from build123d import *

# Parameters (mm, degrees)
SALIENTE_EXTRUIR1_DEPTH = 11
REDONDEO1_R             = 5
REDONDEO2_R             = 3
CROQUIS2_R              = 2.5
SALIENTE_EXTRUIR2_DEPTH = 11
CROQUIS3_W              = 8
CROQUIS3_H              = 15
CORTAR_EXTRUIR1_DEPTH   = 15
CROQUIS4_W              = 1.857543752
CROQUIS4_H              = 12.596468565
SALIENTE_EXTRUIR3_DEPTH = 13


with BuildPart() as part:
    # Croquis1 → Saliente-Extruir1 (new body)
    with BuildSketch(Plane.XY):
        Polygon((0, 9.6), (0, -9.6), (-32, -9), (-32, 9), align=None)
    extrude(amount=SALIENTE_EXTRUIR1_DEPTH)

    # Redondeo1
    redondeo1_edges = [part.edges().sort_by_distance(p)[0] for p in [
        (-32, -9, 5.5),
        (-32, 9, 5.5),
    ]]
    fillet(redondeo1_edges, radius=REDONDEO1_R)

    # Redondeo2
    redondeo2_edges = [part.edges().sort_by_distance(p)[0] for p in [
        (-13.546866762, 9.345996248, 11),
        (-13.546866762, -9.345996248, 0),
        (-13.546866762, -9.345996248, 11),
        (-32, 0, 0),
        (-30.568519835, 7.595108483, 0),
        (-30.568519835, -7.595108483, 0),
        (-32, 0, 11),
        (-30.568519835, 7.595108483, 11),
        (-30.568519835, -7.595108483, 11),
        (-13.546866762, 9.345996248, 0),
    ]]
    fillet(redondeo2_edges, radius=REDONDEO2_R)

    # Croquis2 → Saliente-Extruir2 (add)
    with BuildSketch(Plane.ZY.offset(32)):
        with Locations((5.5, 0)):
            Circle(CROQUIS2_R)
    extrude(amount=SALIENTE_EXTRUIR2_DEPTH)

    # Croquis3 → Cortar-Extruir1 (cut)
    with BuildSketch(Plane(origin=(0, 0, 0), x_dir=(0, 0, -1), z_dir=(1, 0, 0))):
        with Locations((-5.5, 0)):
            Rectangle(CROQUIS3_W, CROQUIS3_H)
    extrude(amount=-CORTAR_EXTRUIR1_DEPTH, mode=Mode.SUBTRACT)

    # Croquis4 → Saliente-Extruir3 (add)
    with BuildSketch(Plane(origin=(-15, 0, 0), x_dir=(0, 0, -1), z_dir=(1, 0, 0))):
        with Locations((-6.633221346, -0.002349923)):
            Rectangle(CROQUIS4_W, CROQUIS4_H)
    extrude(amount=SALIENTE_EXTRUIR3_DEPTH)


solid = part.part
Can you work these out from the model? Positions are in its coordinate system, mm. A direction names the side the tool comes from. Coordinates: 2 decimals unless noted, no trailing zeros. Loops run counter-clockwise (first coordinate to the right, second up) from the corner with the lowest first, then second, coordinate; pieces in that order, holes last. Notation, with made-up numbers: (41.25, 54.25) - (78.25, 54.25) arc R13 ccw to (78.25, 62.25) - close; hole circle Ø3 at (-23.5, 29.25). An arc over 180 degrees is marked (long way). Answer as a JSON object with one key per item and string values. Group by question number.
Item 1: If I drill on L1, parallel to Z at x = -6, y = -5; L2, parallel to Y at x = -7, z = 6; L3, parallel to Y at x = -7, z = 3.5, over which ranges is the centre line in solid material (lowest first)? Write a range as from..to.
Item 2: If we mould it in two halves opening along Z, with no side actions, what happens to faces 4 (the face through (-14, 0, 0)), 5 (the face through (-2, 0, 7)), 6 (the face through (-43, 0, 5))? For each: released by +Z, released by -Z, zero draft, split by the parting line, or undercut.
Item 3: For pin 1 (2.5 mm diameter, centred on x = -9, z = 4.5, fed in from +Y); pin 2 (5 mm diameter, centred on y = 7.5, z = 2.5, fed in from -X); pin 3 (2 mm diameter, centred on x = -11, z = 6.5, fed in from -Y); pin 4 (5 mm diameter, centred on x = -37, y = 6, fed in from -Z), each with a flat end and sliding along its axis, tell me the tip position at first contact or that it passes through.
Item 4: On a 3-axis mill with a long thin cutter (end or side, diameter ignored), from which of +Z, -Z, +X, -X, +Y, -Y can I reach the whole of each face in a straight line? I mean faces 1 (the face through (-13.34, 8.49, 0.9)), 2 (the face through (-9, 0, 7.562)), 3 (the face through (-13.72, -8.44, 10.145)). Say none if no direction works.
Item 5: If we section it at B-B (x = -9): State how many separate pieces and enclosed holes the cut face has, plus the area to 3 significant figures.
Item 6: If we section it at A-A (y = 1.5): List the corners of the cut face in (x, z) for me, plus the area to 3 significant figures.
Item 7: If we section it at D-D (x = -38.5): List the corners of the cut face in (y, z) for me.
Item 8: If we section it at C-C (z = 6.5): List the corners of the cut face in (x, y) for me, plus the area to 3 significant figures.
Returned:
{
 "1": {"L1": "z = 0..1.5, 5.7..7.56, 9.5..11", "L2": "y = -9.47..-7.5, -6.3..6.3, 7.5..9.47", "L3": "y = -9.47..-7.5, 7.5..9.47"},
 "2": {"face 4": "released by -Z", "face 5": "undercut", "face 6": "zero draft"},
 "3": {"pin 1": "stops at y = 9.45", "pin 2": "stops at x = -31.91", "pin 3": "stops at y = -9.41", "pin 4": "passes through"},
 "4": {"face 1": "-Z, -X, +Y", "face 2": "+X", "face 3": "+Z, -X, -Y"},
 "5": {"separate pieces": "2", "enclosed holes": "1", "area": "103 mm²"},
 "6": {"outline": "(-43, 3.5) - (-32, 3.5) - (-32, 3) arc R3 ccw to (-29, 0) - (0, 0) - (0, 1.5) - (-15, 1.5) - (-15, 5.7) - (-2, 5.7) - (-2, 7.56) - (-15, 7.56) - (-15, 9.5) - (0, 9.5) - (0, 11) - (-29, 11) arc R3 ccw to (-32, 8) - (-32, 7.5) - (-43, 7.5) - close", "area": "296 mm²"},
 "7": {"outline": "circle Ø5 at (0, 5.5)"},
 "8": {"outline": "(-43, -2.29) - (-32, -2.29) - (-32, -4.09) arc R5 ccw to (-27.09, -9.09) - (0, -9.6) - (0, -7.5) - (-15, -7.5) - (-15, -6.3) - (-2, -6.3) - (-2, 6.3) - (-15, 6.3) - (-15, 7.5) - (0, 7.5) - (0, 9.6) - (-27.09, 9.09) arc R5 ccw to (-32, 4.09) - (-32, 2.29) - (-43, 2.29) - close", "area": "574 mm²"}
}
